Autodesk Inventor part; units mm, degrees
ref_plane "YZ Plane" through (0, 0, 0) normal (1, 0, 0) x (0, 1, 0)
ref_plane "XZ Plane" through (0, 0, 0) normal (0, 1, 0) x (-1, 0, 0)
ref_plane "XY Plane" through (0, 0, 0) normal (0, 0, 1) x (1, 0, 0)
sketch "Sketch1" plane through (0, 0, 0) normal (0, 0, 1) x (1, 0, 0)
  line L0 (0, 0) -> (0, 17.5) construction
  line L1 (0, 0) -> (-10, 0)
  line L2 (0, 0) -> (10, 0)
  line L3 (-10, 0) -> (-10, 4.6)
  line L4 (-10, 4.6) -> (-6.1, 8.5)
  line L5 (-6.1, 8.5) -> (-6.1, 9)
  line L6 (-6.1, 9) -> (-10, 12.9)
  line L7 (-10, 12.9) -> (-10, 15.4)
  line L8 (-10, 15.4) -> (-7.9, 17.5)
  line L9 (-7.9, 17.5) -> (0, 17.5)
  line L10 (10, 0) -> (10, 4.6)
  line L11 (10, 4.6) -> (6.1, 8.5)
  line L12 (6.1, 8.5) -> (6.1, 9)
  line L13 (6.1, 9) -> (10, 12.9)
  line L14 (10, 12.9) -> (10, 15.4)
  line L15 (10, 15.4) -> (7.9, 17.5)
  line L16 (7.9, 17.5) -> (0, 17.5)
  dimension "d0" = 17.5
  dimension "d1" = 20
  dimension "d2" = 4.6
  dimension "d3" = 8.5
  dimension "d8" = 135
  dimension "d9" = 0.5
  dimension "d10" = 135
  dimension "d11" = 2.5
extrude "Extrusion1" add sketch "Sketch1" along normal blind 400
sketch "Sketch2" plane through (0, 0, 0) normal (0, 1, 0) x (-1, 0, 0)
  line L0 (0, 0) -> (0, 20) construction
  line L1 (0, 20) -> (0, 80) construction
  circle A0 centre (0, 20) radius 4.75
  circle A1 centre (0, 20) radius 3
  dimension "d14" = 20
  dimension "d15" = 60
  dimension "d16" = 9.5
  dimension "d17" = 6
extrude "Extrusion2" cut sketch "Sketch2" along normal through all contours A1
extrude "Extrusion3" cut sketch "Sketch2" against normal blind 8.5 from surface at 17.5
pattern_linear "Rectangular Pattern1" count 9 spacing 60 along (0, 0, 1) of "Extrusion2", "Extrusion3"
properties part number "HGR20 400mm"
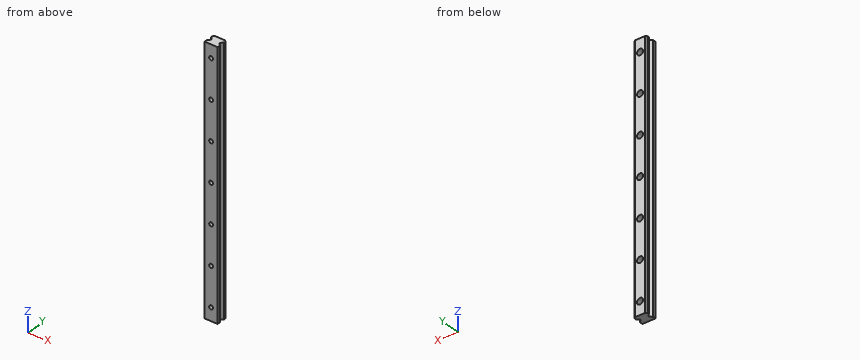
Here's how the part is built. I have some questions about the finished solid (model axes, mm). Give positions to 0.01 mm unless a question says otherwise; leave off trailing zeros. Order: outer loops, then holes, each group sorted by start corner. A loop starts at its lowest first (then second) coordinate and runs counter-clockwise, first axis right, second up. Notation, with made-up numbers: M -6,76.5 L 6,76.5 A19 ccw 6,110.5 Z; hole C -30,46.25 d2. An arc over 180 degrees is marked long. Use a Markdown table: item, result. Add a question column.
1. For pin 1 Ø8.5 at (x, z) = (0, 20) entering from +Y; pin 2 Ø5 at (y, z) = (9.5, 322.5) entering from +X; pin 3 Ø5.5 at (x, z) = (0, 200) entering from -Y, each with a flat end and sliding along its axis, tell me the tip position at first contact or that it passes through.
2. Suppose I cut it at A-A (z = 212). List the corners of the cut face in (x, y) for me, and give its area (3 significant figures).
3. I need wall thicknesses on probe 1 along X at (y, z) = (3.25, 200); probe 2 along Y at (x, z) = (-8.5, 160); probe 3 along Y at (x, z) = (-6.75, 243). Which ranges of each line are inside material? Lowest first, please. Write a range as from..to.
Results list:
| question | item | result |
|---|---|---|
| 1 | pin 1 | stops at y = 9 |
| 1 | pin 2 | stops at x = 9.1 |
| 1 | pin 3 | passes through |
| 2 | outline | M -10,0 L 10,0 L 10,4.6 L 6.1,8.5 L 6.1,9 L 10,12.9 L 10,15.4 L 7.9,17.5 L -7.9,17.5 L -10,15.4 L -10,12.9 L -6.1,9 L -6.1,8.5 L -10,4.6 Z |
| 2 | area | 311 mm² |
| 3 | probe 1 | x = -10..-3, 3..10 |
| 3 | probe 2 | y = 0..6.1, 11.4..16.9 |
| 3 | probe 3 | y = 0..7.85, 9.65..17.5 |
